from build123d import *

# Parameters (mm, degrees)
SKETCH1_W         = 44.38767267
SKETCH1_H         = 8.89569146
EXTRUDE1_DEPTH    = 1.905
SKETCH2_R         = 4.2291
SKETCH2_R_2       = 2.9718
EXTRUDE2_DEPTH    = 3.0226
LPATTERN2_COUNT   = 5
LPATTERN2_PITCH   = 2.54
CIRPATTERN2_COUNT = 2


with BuildPart() as part:
    # Sketch1 → Extrude1 (new body)
    with BuildSketch(Plane.XY):
        Rectangle(SKETCH1_W, SKETCH1_H)
    extrude(amount=EXTRUDE1_DEPTH)

    # Sketch2 → Extrude2 (add)
    with BuildSketch(Plane(origin=(0, 0, 0), x_dir=(-1, 0, 0), z_dir=(0, 0, -1))):
        Circle(SKETCH2_R)
        Circle(SKETCH2_R_2, mode=Mode.SUBTRACT)
    extrude(amount=EXTRUDE2_DEPTH)

    # Sketch4 → #53 (0.0595) Diameter Hole1 (revolve, cut)
    with BuildSketch(Plane(origin=(6.985, 0, 1.905), x_dir=(0, -1, 0), z_dir=(1, 0, 0))):
        Polygon((0, 0), (0, 5.534040327), (0.75565, 5.08), (0.75565, 0), align=None)
    f_53_0_0595_diameter_hole1 = revolve(axis=Axis((6.985, 0, 8.255), (0, 0, -1)), mode=Mode.SUBTRACT)

    # LPattern2: #53 (0.0595) Diameter Hole1 ×5
    with Locations(*[(i * LPATTERN2_PITCH, 0, 0) for i in range(1, LPATTERN2_COUNT)]):
        add(f_53_0_0595_diameter_hole1, mode=Mode.SUBTRACT)

    # CirPattern2: #53 (0.0595) Diameter Hole1 ×2 about axis
    cirpattern2_axis = Axis((0, 0, 0), (0, 0, 1))
    for i in range(1, CIRPATTERN2_COUNT):
        add(f_53_0_0595_diameter_hole1.rotate(cirpattern2_axis, i * 360 / CIRPATTERN2_COUNT), mode=Mode.SUBTRACT)

    # CirPattern2 copy 1 sketch → CirPattern2 copy 1 (revolve, cut)
    with BuildSketch(Plane(origin=(-9.525, 0, 1.905), x_dir=(0, 1, 0), z_dir=(-1, 0, 0))):
        Polygon((0, 0), (0, 5.534040327), (0.75565, 5.08), (0.75565, 0), align=None)
    revolve(axis=Axis((-9.525, 0, 8.255), (0, 0, -1)), mode=Mode.SUBTRACT)

    # CirPattern2 copy 2 sketch → CirPattern2 copy 2 (revolve, cut)
    with BuildSketch(Plane(origin=(-12.065, 0, 1.905), x_dir=(0, 1, 0), z_dir=(-1, 0, 0))):
        Polygon((0, 0), (0, 5.534040327), (0.75565, 5.08), (0.75565, 0), align=None)
    revolve(axis=Axis((-12.065, 0, 8.255), (0, 0, -1)), mode=Mode.SUBTRACT)

    # CirPattern2 copy 3 sketch → CirPattern2 copy 3 (revolve, cut)
    with BuildSketch(Plane(origin=(-14.605, 0, 1.905), x_dir=(0, 1, 0), z_dir=(-1, 0, 0))):
        Polygon((0, 0), (0, 5.534040327), (0.75565, 5.08), (0.75565, 0), align=None)
    revolve(axis=Axis((-14.605, 0, 8.255), (0, 0, -1)), mode=Mode.SUBTRACT)

    # CirPattern2 copy 4 sketch → CirPattern2 copy 4 (revolve, cut)
    with BuildSketch(Plane(origin=(-17.145, 0, 1.905), x_dir=(0, 1, 0), z_dir=(-1, 0, 0))):
        Polygon((0, 0), (0, 5.534040327), (0.75565, 5.08), (0.75565, 0), align=None)
    revolve(axis=Axis((-17.145, 0, 8.255), (0, 0, -1)), mode=Mode.SUBTRACT)


solid = part.part
Source: CAD feature listing. Evaluate the final solid. Frame: model axes, mm. A direction names the side the tool comes from. Round coordinates to 2 decimals unless told otherwise and drop trailing zeros. Loops run counter-clockwise (first coordinate to the right, second up) from the corner with the lowest first, then second, coordinate; pieces in that order, holes last. Notation, with made-up numbers: (-33.5, 77.5) - (-16.5, 77.5) arc R9 cw to (-16.5, 84.5) - close; hole circle Ø5 at (83, -34). An arc over 180 degrees is marked (long way). Write item = value, one per line. Start each with the question number.
Item 1: Section query D-D on z = -1.9. Output: boundary loops of the cut face in (x, y).
Item 2: Reachability of faces 1 (the face through (0.917, -4.129, -1.49)), 2 (the face through (-10.263, -0.164, 0.966)) from +Z, -Z, +X, -X, +Y, -Y: full face, straight path, thin tool, end or side. Return the list, or none.
Item 3: Section query C-C on y = 0. Count the separate pieces of the cut face and the enclosed holes in it, plus the area to 3 significant figures.
Item 4: Section query A-A on x = 0. Output: boundary loops of the cut face in (y, z) (3 decimals).
Item 5: Mould query, pull axis X, two halves, no side actions, for faces 3 (the face through (6.236, 0.098, 0.966)), 4 (the face through (-22.194, 0, 1)), 5 (the face through (22.194, 0, 1)), 6 (the face through (10.263, 0.164, 0.966)). Classes: released by +X, released by -X, zero draft, split by the parting line, or undercut.
Item 6: Material intervals for line 1 (Y direction, x = 14.5, z = 1.45); line 2 (Z direction, x = 12, y = 3) (3 decimals); line 3 (X direction, y = 0.75, z = -0.3), sorted ascending.
Item 7: First-contact query: pin 1 Ø0.9 at (x, y) = (-9.525, 0) entering from +Z; pin 2 Ø2.5 at (x, y) = (14.605, 0) entering from -Z. Flat tips, straight axial feed; report the tip coordinate or a pass-through.
Item 8: Section query B-B on y = -3.75. Output: boundary loops of the cut face in (x, z) (3 decimals).
Results list:
q1.outline = circle Ø8.46 at (0, 0); hole circle Ø5.94 at (0, 0)
q2.face_1 = -Z
q2.face_2 = +Z, -Z
q3.separate_pieces = 11
q3.enclosed_holes = 0
q3.area = 63.4 mm²
q4.outline = (-4.448, 0) - (-4.229, 0) - (-4.229, -3.023) - (-2.972, -3.023) - (-2.972, 0) - (2.972, 0) - (2.972, -3.023) - (4.229, -3.023) - (4.229, 0) - (4.448, 0) - (4.448, 1.905) - (-4.448, 1.905) - close
q5.face_3 = undercut
q5.face_4 = released by -X
q5.face_5 = released by +X
q5.face_6 = undercut
q6.line_1 = -4.45 to -0.75, 0.75 to 4.45
q6.line_2 = 0 to 1.905
q6.line_3 = -4.16 to -2.88, 2.88 to 4.16
q7.pin_1 = through
q7.pin_2 = 0
q8.outline = (-22.194, 0) - (-1.955, 0) - (-1.955, -3.023) - (1.955, -3.023) - (1.955, 0) - (22.194, 0) - (22.194, 1.905) - (-22.194, 1.905) - close
